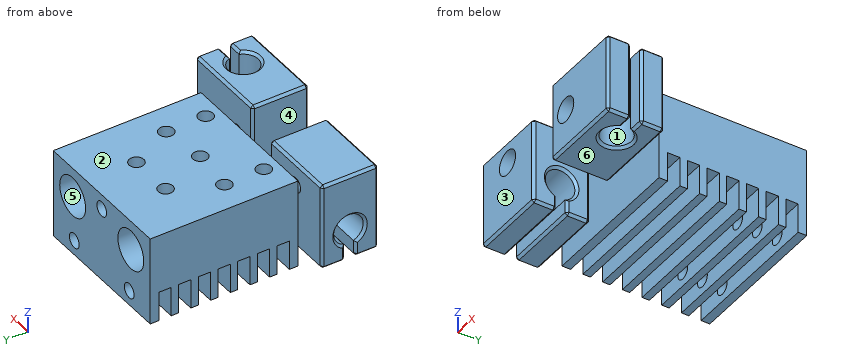
```python
from build123d import *

# Parameters (mm, degrees)
F0_W      = 30
F0_H      = 30
F11_DEPTH = 18
F1_D      = 8
F1_DEPTH  = 6.5
F1_TIP    = 2.4034424761
F13_W     = 30
F13_H     = 2.5
F14_DEPTH = 6
F15_D     = 3
F15_DEPTH = 10
F15_TIP   = 0.9012909285
F2_R      = 1.475
F3_DEPTH  = 3.5
F17_W     = 16
F17_H     = 17.5
F16_W     = 17.5
F16_H     = 16
F18_DEPTH = 11.5
F5_DEPTH  = 16
F21_DEPTH = 16
F8_SIZE   = 0.5
F7_R      = 1.5
F9_DEPTH  = 8
F20_R     = 2.5
F19_R     = 2.5
F10_DEPTH = 6


# Not quite as in the source:
# - a feature names something its author has since deleted; it is built from what else it names


with BuildPart() as f11:
    # F0 (on Top) → F11 (new body)
    with BuildSketch(Plane.XY):
        Rectangle(F0_W, F0_H)
    extrude(amount=F11_DEPTH)

    # F1
    with Locations(Plane(origin=(0, 15, 0), x_dir=(-1, 0, 0), z_dir=(0, 1, 0))):
        with Locations((-9, 12), (9, 12)):
            Hole(F1_D / 2, depth=F1_DEPTH)
            with Locations((0, 0, -(F1_DEPTH + F1_TIP / 2))):  # 118° drill point
                Cone(0, F1_D / 2, F1_TIP, mode=Mode.SUBTRACT)

    # F13 (on face) → F14 (cut)
    with BuildSketch(Plane(origin=(0, 0, 0), x_dir=(1, 0, 0), z_dir=(0, 0, -1))):
        with Locations((0, 12)):
            Rectangle(F13_W, F13_H)
        with Locations((0, 8)):
            Rectangle(F13_W, F13_H)
        with Locations((0, 4)):
            Rectangle(F13_W, F13_H)
        Rectangle(F13_W, F13_H)
        with Locations((0, -4)):
            Rectangle(F13_W, F13_H)
        with Locations((0, -8)):
            Rectangle(F13_W, F13_H)
        with Locations((0, -12)):
            Rectangle(F13_W, F13_H)
    extrude(amount=-F14_DEPTH, mode=Mode.SUBTRACT)

    # F15
    with Locations(Plane(origin=(0, 15, 0), x_dir=(-1, 0, 0), z_dir=(0, 1, 0))):
        with Locations((8.5, 3), (-8.5, 3), (0, 15)):
            Hole(F15_D / 2, depth=F15_DEPTH)
            with Locations((0, 0, -(F15_DEPTH + F15_TIP / 2))):  # 118° drill point
                Cone(0, F15_D / 2, F15_TIP, mode=Mode.SUBTRACT)

    # F2 (on face) → F3 (join)
    with BuildSketch(Plane.XZ.offset(15)):
        with Locations((-9, 12)):
            Circle(F2_R)
        with Locations((9, 12)):
            Circle(F2_R)
    extrude(amount=F3_DEPTH)

    # F17 (on face) + F16 (on face) → F18 (join)
    with BuildSketch(Plane.XZ.offset(18.5)):
        with Locations((-9, 7.75)):
            Rectangle(F17_W, F17_H)
    with BuildSketch(Plane.XZ.offset(18.5)):
        with Locations((13.25, 12)):
            Rectangle(F16_W, F16_H)
    extrude(amount=F18_DEPTH)

    # F4 (on face) → F5 (cut, through all)
    with BuildSketch(Plane(origin=(0, 0, 4), x_dir=(1, 0, 0), z_dir=(0, 0, -1))):
        with BuildLine():
            Line((22, 25.25), (18.8284271247, 25.25))
            ThreePointArc((18.8284271247, 25.25), (13, 24.25), (18.8284271247, 23.25))
            Line((18.8284271247, 23.25), (22, 23.25))
            Line((22, 23.25), (22, 25.25))
        make_face()
    extrude(amount=-F5_DEPTH, mode=Mode.SUBTRACT)

    # F6 (on face) → F21 (cut, through all)
    with BuildSketch(Plane(origin=(-17, 0, 0), x_dir=(0, -1, 0), z_dir=(-1, 0, 0))):
        with BuildLine():
            Line((25.25, -1), (25.25, 2.1715728753))
            ThreePointArc((25.25, 2.1715728753), (24.25, 8), (23.25, 2.1715728753))
            Line((23.25, 2.1715728753), (23.25, -1))
            Line((23.25, -1), (25.25, -1))
        make_face()
    extrude(amount=-F21_DEPTH, mode=Mode.SUBTRACT)

    # F8
    f8_edges = [f11.edges().sort_by_distance(p)[0] for p in [
        (13.25, -18.5, 4),
        (22, -20.875, 4),
        (20.414214, -23.25, 4),
        (13, -24.25, 4),
        (20.414214, -25.25, 4),
        (22, -27.625, 4),
        (13.25, -30, 4),
        (4.5, -24.25, 4),
        (4.5, -24.25, 20),
        (4.5, -18.5, 12),
        (4.5, -30, 12),
        (-9, -25.25, -1),
        (-1, -27.625, -1),
        (-9, -30, -1),
        (-17, -27.625, -1),
        (-9, -18.5, -1),
        (-1, -20.875, -1),
        (-9, -23.25, -1),
        (-17, -20.875, -1),
        (-1, -18.5, 7.75),
        (-1, -24.25, 16.5),
        (-1, -30, 7.75),
        (-1, -25.25, 0.585786),
        (-1, -24.25, 8),
        (-1, -23.25, 0.585786),
        (22, -18.5, 12),
        (22, -20.875, 20),
        (22, -23.25, 12),
        (22, -25.25, 12),
        (22, -27.625, 20),
        (22, -30, 12),
        (-17, -24.25, 16.5),
        (-9, -18.5, 16.5),
        (-9, -30, 16.5),
        (-17, -18.5, 7.75),
        (-17, -23.25, 0.585786),
        (-17, -24.25, 8),
        (-17, -25.25, 0.585786),
        (-17, -30, 7.75),
        (13.25, -18.5, 20),
        (13.25, -30, 20),
        (20.414214, -25.25, 20),
        (13, -24.25, 20),
        (20.414214, -23.25, 20),
    ]]
    chamfer(f8_edges, length=F8_SIZE)

    # F7 (on face) → F9 (cut)
    with BuildSketch(Plane.XY.offset(18)):
        with Locations((-9, -12)):
            Circle(F7_R)
        with Locations((-9, -4)):
            Circle(F7_R)
        with Locations((0, -5)):
            Circle(F7_R)
        with Locations((4.5, 5)):
            Circle(F7_R)
        with Locations((9, -4)):
            Circle(F7_R)
        with Locations((9, -12)):
            Circle(F7_R)
        with Locations((-4.5, 5)):
            Circle(F7_R)
    extrude(amount=-F9_DEPTH, mode=Mode.SUBTRACT)

    # F20 (on face) + F19 (on face) → F10 (cut)
    with BuildSketch(Plane.XZ.offset(30)):
        with Locations((-9, 12)):
            Circle(F20_R)
    with BuildSketch(Plane.XZ.offset(30)):
        with Locations((9, 12)):
            Circle(F19_R)
    extrude(amount=-F10_DEPTH, mode=Mode.SUBTRACT)


solid = f11.part
```
Check sheet for the modelled part. Datum: model origin and axes. Units: mm. Face numbers are marked on the shaded views. A direction names the side the tool comes from. Give positions to 0.01 mm unless a question says otherwise; leave off trailing zeros. Loops run counter-clockwise (first coordinate to the right, second up) from the corner with the lowest first, then second, coordinate; pieces in that order, holes last. Notation, with made-up numbers: M -3.75,26 L 10.25,26 A35 ccw 10.25,61 Z; hole C 74,63.25 d2. An arc over 180 degrees is marked long. Answer in a Markdown table with one row per item.
1) Mould release check, pull along Y, two halves, no side actions. Record for the marked faces 1, 2 and 3: released by +Y, released by -Y, zero draft, split by the parting line, or undercut.
Solutions:
| item | result |
|---|---|
| face 1 | undercut |
| face 2 | zero draft |
| face 3 | released by -Y |
2) Cross-section at C-C (y = 11.5). Enter the section's corners in (x, z), plus the area to 3 significant figures.
Solutions:
| item | result |
|---|---|
| outline | M -15,6 L 15,6 L 15,18 L -15,18 Z; hole C -9,12 d8; hole C 0,15 d3; hole C 9,12 d8 |
| area | 252 mm^2 |
3) Depth check by flat-ended pin: pin 1 (5 mm diameter, centred on y = -6.5, z = 15.5, fed in from -X); pin 2 (0.8 mm diameter, centred on x = 20.5, z = 12, fed in from +Y); pin 3 (3 mm diameter, centred on x = 9, z = 12, fed in from +Y). Enter the tip coordinate at first touch or a pass-through.
Solutions:
| item | result |
|---|---|
| pin 1 | stops at x = -15 |
| pin 2 | stops at y = -18.5 |
| pin 3 | stops at y = 7 |
4) Thickness scan on line 1 (Z direction, x = 0, y = 10); line 2 (Z direction, x = 9, y = -25); line 3 (Z direction, x = -9.5, y = -26). Record the ranges inside material, lowest first.
Solutions:
| item | result |
|---|---|
| line 1 | z = 0 to 13.5, 16.5 to 18 |
| line 2 | z = 4 to 9.5, 14.5 to 20 |
| line 3 | z = -1 to 2.56, 7.44 to 9.55, 14.45 to 16.5 |
5) Cross-section at B-B (y = -20). Enter the section's corners in (x, z).
Solutions:
| item | result |
|---|---|
| outline | M -17,-0.5 L -16.5,-1 L -1.5,-1 L -1,-0.5 L -1,16 L -1.5,16.5 L -16.5,16.5 L -17,16 Z; M 4.5,4.5 L 5,4 L 21.5,4 L 22,4.5 L 22,19.5 L 21.5,20 L 5,20 L 4.5,19.5 Z |
6) Cross-section at A-A (x = 16). Enter the section's corners in (y, z).
Solutions:
| item | result |
|---|---|
| outline | M -30,4.5 L -29.5,4 L -27.75,4 L -27.25,4.5 L -27.25,19.5 L -27.75,20 L -29.5,20 L -30,19.5 Z; M -21.25,4.5 L -20.75,4 L -19,4 L -18.5,4.5 L -18.5,19.5 L -19,20 L -20.75,20 L -21.25,19.5 Z |
7) Tool access check on the marked faces 4, 5 and 6. Record the directions out of +Z, -Z, +X, -X, +Y, -Y that give a thin tool (end or side, any length) a straight path to the whole face; none if there is none.
Solutions:
| item | result |
|---|---|
| face 4 | +Z, -Z, -Y |
| face 5 | +Y |
| face 6 | -Z, +X, -Y |
